Autodesk Inventor part; units mm, degrees
ref_plane "YZ Plane" through (0, 0, 0) normal (1, 0, 0) x (0, 1, 0)
ref_plane "XZ Plane" through (0, 0, 0) normal (0, 1, 0) x (-1, 0, 0)
ref_plane "XY Plane" through (0, 0, 0) normal (0, 0, 1) x (1, 0, 0)
sketch "Sketch2" plane through (0, 0, 0) normal (0, 0, 1) x (1, 0, 0)
  line L0 (0, 0) -> (73, 0)
  line L1 (73, 0) -> (73, 73)
  line L2 (73, 73) -> (0, 73)
  line L3 (0, 73) -> (0, 0)
  dimension "d2" = 73
  dimension "d3" = 73
extrude "Extrusion1" add sketch "Sketch2" along normal blind 20
sketch "Sketch3" plane through (0, 0, 0) normal (0, 0, -1) x (-1, 0, 0)
  line L0 (-73, 73) -> (0, 73)
  line L1 (0, 73) -> (0, 0)
  line L2 (-73, 73) -> (0, 73)
  line L3 (0, 73) -> (0, 0)
  line L4 (0, 0) -> (-73, 0)
  line L5 (-73, 0) -> (-73, 73)
  line L6 (-69, 69) -> (-4, 69)
  line L7 (-4, 69) -> (-4, 4)
  line L8 (-4, 4) -> (-69, 4)
  line L9 (-69, 4) -> (-69, 69)
  dimension "d6" = 4
extrude "Extrusion2" cut sketch "Sketch3" against normal blind 20 contours L6 L7 L8 L9
sketch "Sketch4" plane through (0, 0, 20) normal (0, 0, 1) x (1, 0, 0)
  line L0 (4, 4) -> (4, 69)
  line L1 (69, 69) -> (69, 4)
  line L2 (4, 4) -> (69, 4)
  line L3 (69, 4) -> (69, 69)
  line L4 (69, 69) -> (4, 69)
  line L5 (4, 69) -> (4, 4)
  line L6 (5, 68) -> (68, 68)
  line L7 (68, 68) -> (68, 5)
  line L8 (68, 5) -> (5, 5)
  line L9 (5, 5) -> (5, 68)
  point P0 (0, 0)
  point P1 (69, 4)
  point P2 (4, 69)
  dimension "d9" = 1
extrude "Extrusion3" add sketch "Sketch4" against normal blind 1
sketch "Sketch5" plane through (0, 0, 0) normal (0, 0, -1) x (-1, 0, 0)
  line L0 (-4, 69) -> (-4, 4)
  line L1 (-4, 4) -> (-69, 4)
  line L2 (-4, 69) -> (-69, 69)
  line L3 (-69, 69) -> (-69, 4)
  line L4 (-69, 4) -> (-4, 4)
  line L5 (-4, 4) -> (-4, 69)
  line L6 (0, 73) -> (0, 0)
  line L7 (0, 0) -> (-73, 0)
  line L8 (0, 73) -> (-73, 73)
  line L9 (-73, 73) -> (-73, 0)
  line L10 (-73, 0) -> (0, 0)
  line L11 (0, 0) -> (0, 73)
extrude "Extrusion4" add sketch "Sketch5" along normal blind 13.5
sketch "Sketch7" plane through (73, 0, 20) normal (1, 0, 0) x (0, 0, -1)
  line L0 (33.5, 69) -> (33.5, 4)
  line L1 (29.6, 36.5) -> (29.6, 51.5)
  line L2 (29.6, 51.5) -> (15.6, 51.5)
  line L3 (15.6, 51.5) -> (15.6, 21.5)
  line L4 (15.6, 21.5) -> (29.6, 21.5)
  line L5 (29.6, 21.5) -> (29.6, 36.5)
  point P0 (20, 0)
  dimension "d43" = 15
  dimension "d44" = 14
  dimension "d45" = 30
extrude "Extrusion5" cut sketch "Sketch7" against normal blind 4
sketch "Sketch8" plane through (0, 0, 20) normal (-1, 0, 0) x (0, 0, 1)
  circle A0 centre (-24, 65) radius 2.5
  point P0 (-20, 0)
  point P1 (-33.5, 69)
  dimension "d106" = 5
extrude "Extrusion6" cut sketch "Sketch8" against normal blind 4
sketch "Sketch10" plane through (0, 73, 20) normal (0, 1, 0) x (1, 0, 0)
  line L0 (0, 0) -> (73, 0)
  line L1 (73, 33.5) -> (0, 33.5)
  line L2 (0, 33.5) -> (0, 0)
  line L3 (4, 33.5) -> (4, 1)
  line L4 (51.2, 20.4) -> (47.2, 20.4)
  line L5 (47.2, 20.4) -> (47.2, 16.4)
  line L6 (47.2, 16.4) -> (42.8, 16.4)
  line L7 (42.8, 16.4) -> (42.8, 20.4)
  line L8 (42.8, 20.4) -> (38.8, 20.4)
  line L9 (38.8, 20.4) -> (38.8, 24.8)
  line L10 (38.8, 24.8) -> (42.8, 24.8)
  line L11 (42.8, 24.8) -> (42.8, 28.8)
  line L12 (42.8, 28.8) -> (47.2, 28.8)
  line L13 (47.2, 28.8) -> (47.2, 24.8)
  line L14 (47.2, 24.8) -> (51.2, 24.8)
  line L15 (51.2, 24.8) -> (51.2, 20.4)
  line L16 (24.8, 20.4) -> (37.2, 20.4)
  line L17 (37.2, 20.4) -> (37.2, 24.8)
  line L18 (37.2, 24.8) -> (24.8, 24.8)
  line L19 (24.8, 24.8) -> (24.8, 20.4)
  line L20 (10.161, 22.4041) -> (23.2, 28.9236)
  line L21 (23.2, 28.9236) -> (23.2, 15.8846)
  line L22 (23.2, 15.8846) -> (10.161, 22.4041)
  line L23 (23.1, 28.7618) -> (10.3846, 22.4041)
  line L24 (10.3846, 22.4041) -> (23.1, 16.0464)
  line L25 (23.1, 16.0464) -> (23.1, 28.7618)
  line L26 (24.9, 24.7) -> (37.1, 24.7)
  line L27 (37.1, 24.7) -> (37.1, 20.5)
  line L28 (37.1, 20.5) -> (24.9, 20.5)
  line L29 (24.9, 20.5) -> (24.9, 24.7)
  line L30 (42.9, 24.7) -> (38.9, 24.7)
  line L31 (38.9, 24.7) -> (38.9, 20.5)
  line L32 (38.9, 20.5) -> (42.9, 20.5)
  line L33 (42.9, 20.5) -> (42.9, 16.5)
  line L34 (42.9, 16.5) -> (47.1, 16.5)
  line L35 (47.1, 16.5) -> (47.1, 20.5)
  line L36 (47.1, 20.5) -> (51.1, 20.5)
  line L37 (51.1, 20.5) -> (51.1, 24.7)
  line L38 (51.1, 24.7) -> (47.1, 24.7)
  line L39 (47.1, 24.7) -> (47.1, 28.7)
  line L40 (47.1, 28.7) -> (42.9, 28.7)
  line L41 (42.9, 28.7) -> (42.9, 24.7)
  point P0 (0, 20)
  dimension "d95" = 0.1
  dimension "d96" = 0.1
  dimension "d97" = 0.1
extrude "Extrusion8" cut sketch "Sketch10" against normal blind 4 contours L4 L5 L6 L7 L8 L9 L10 L11 L12 L13 L14 L15 | L19 L18 L17 L16 | L20 L21 L22 | L25 L24 L23 | L26 L27 L28 L29 | L41 L40 L39 L38 L37 L36 L35 L34 L33 L32 L31 L30
extrude "Extrusion9" add sketch "Sketch10" against normal blind 4
sketch "Sketch11" plane through (0, 0, 20) normal (-1, 0, 0) x (0, 0, 1)
  circle A0 centre (-24, 65) radius 2.5
  line L0 (-33.5, 4) -> (-33.5, 69)
  line L1 (-33.5, 65) -> (-33.5, 62.5)
  line L2 (-33.5, 62.5) -> (-30.5, 62.5)
  line L3 (-30.5, 62.5) -> (-30.5, 65)
  line L4 (-30.5, 65) -> (-30.5, 67.5)
  line L5 (-30.5, 67.5) -> (-33.5, 67.5)
  line L6 (-33.5, 67.5) -> (-33.5, 65)
  point P0 (-20, 0)
  dimension "d100" = 2.5
  dimension "d101" = 3
  dimension "d102" = 2.5
  dimension "d103" = 2.5
extrude "Extrusion10" cut sketch "Sketch11" against normal blind 3 contours L0 L5 L4 L3 L2
properties part number "Case"
The listing builds one solid part. Answer for the finished solid, in the listing's coordinates (mm). A direction names the side the tool comes from. Coordinates: 2 decimals unless noted, no trailing zeros. Write each loop counter-clockwise with the first axis right and the second up, starting at its lowest first coordinate (ties: lowest second). Pieces come first, ordered by that corner, then holes.
Q1. Which of the six approach directions +Z, -Z, +X, -X, +Y, -Y give full straight-line access (tool end or side, diameter ignored) to faces 3 (the flat face through (36, 0, 3)), 4 (the flat face through (49, 71, -4.7)), 5 (the flat face through (71, 36, -9.6)), 6 (the flat face through (36, 4, 3)), 7 (the flat face through (1, 65, -10.5))?
Returned:
face 3: +Z, -Z, +X, -X, -Y
face 4: +Y
face 5: +X
face 6: -Z
face 7: -Z, -X
Q2. Section C-C, the plane x = 57 is taken. Write down the section's boundary in (y, z), then the cut area to 3 significant figures.
Returned:
outline: (0, -13.5) - (4, -13.5) - (4, 19) - (5, 19) - (5, 20) - (0, 20) - close; (68, 19) - (69, 19) - (69, -13.5) - (73, -13.5) - (73, 20) - (68, 20) - close
area: 270 mm2
Q3. Section A-A, the plane y = 65 is taken. Write down the section's boundary in (x, z).
Returned:
outline: (0, -10.5) - (3, -10.5) - (3, -13.5) - (4, -13.5) - (4, -6.5) - (0, -6.5) - close; (0, -1.5) - (4, -1.5) - (4, 19) - (5, 19) - (5, 20) - (0, 20) - close; (68, 19) - (69, 19) - (69, -13.5) - (73, -13.5) - (73, 20) - (68, 20) - close
Q4. The mould has two halves that part along X. Classify faces 1 (the flat face through (51.1, 71, -3)), 2 (the flat face through (36, 4.6, 20)): released by +X, released by -X, zero draft, split by the parting line, or undercut.
Returned:
face 1: undercut
face 2: zero draft
Q5. Section B-B, the plane x = 44 is taken. Write down the section's boundary in (y, z), then the cut area to 3 significant figures.
Returned:
outline: (0, -13.5) - (4, -13.5) - (4, 19) - (5, 19) - (5, 20) - (0, 20) - close; (68, 19) - (69, 19) - (69, 3.5) - (73, 3.5) - (73, 20) - (68, 20) - close; (69, -13.5) - (73, -13.5) - (73, -8.7) - (69, -8.7) - close
area: 221 mm2
Q6. Find the intervals of material crossed by line 1 along X through (y, z) = (62, 10); line 2 along Y through (x, z) = (2, -4), in increasing order.
Returned:
line 1: x = 0 to 4, 69 to 73
line 2: y = 0 to 62.5, 67.5 to 73
